Job drawing, mm, ordinate dimensions from the low corner. One solid piece. Coordinates: 2 decimals unless noted, no trailing zeros. Write each loop counter-clockwise with the first axis right and the second up, starting at its lowest first coordinate (ties: lowest second). Pieces come first, ordered by that corner, then holes. Notation, with made-up numbers: (-1, -17) - (4, -17) arc R15 ccw to (4, 10) - close; hole circle Ø2 at (47, 50.5). An arc over 180 degrees is marked (long way). Use a Markdown table: item, result.
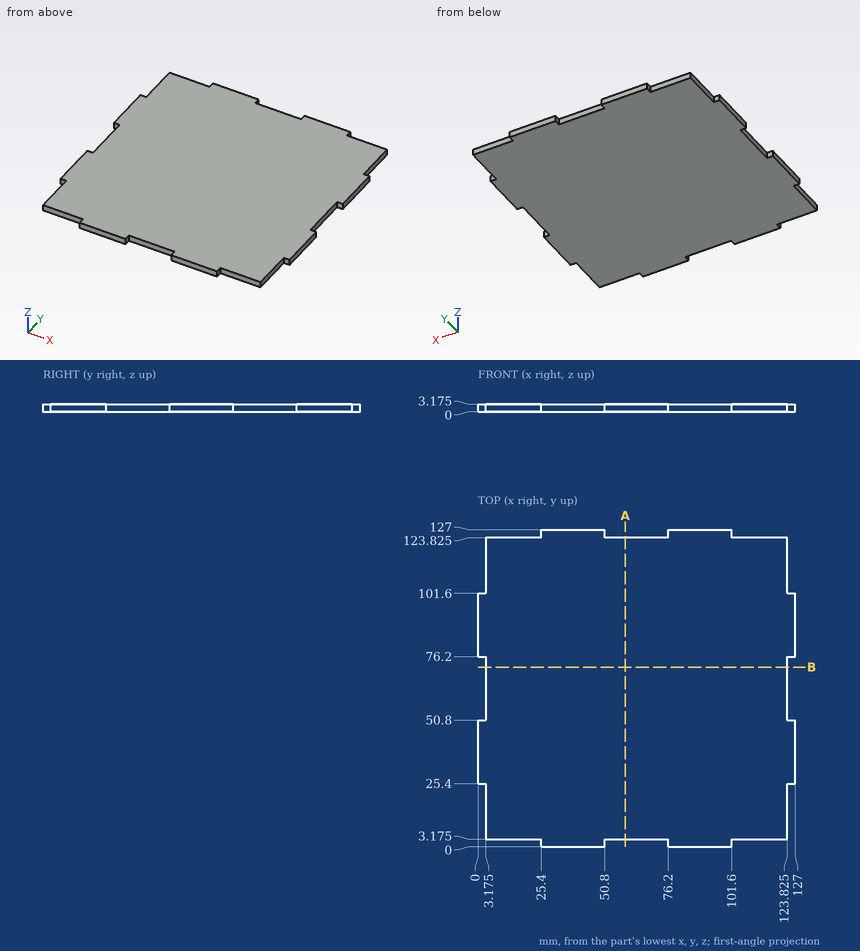
Item 1: Drill centre line: probe 1 along Y at (x, z) = (68, 1.7) (3 decimals). Where is it in solid material? Low to high.
From the geometry:
| item | result |
|---|---|
| probe 1 | 3.175 to 123.825 |
Item 2: Drop flat-ended pins along their axis: P1, Ø1, axis at y = 61.5, z = 1.5, coming from the +X side (3 decimals); P2, Ø1.6, axis at x = 126, z = 1, coming from the -Y side; P3, Ø1.6, axis at x = 64.5, z = 2, coming from the -Y side (3 decimals). Give the stop position or say it passes through.
From the geometry:
| item | result |
|---|---|
| P1 | x = 123.825 |
| P2 | y = 25.4 |
| P3 | y = 3.175 |
Item 3: Band-saw the part on A-A, the plane x = 59. Give the cut face in (y, z) (3 decimals).
From the geometry:
| item | result |
|---|---|
| outline | (3.175, 0) - (123.825, 0) - (123.825, 3.175) - (3.175, 3.175) - close |
